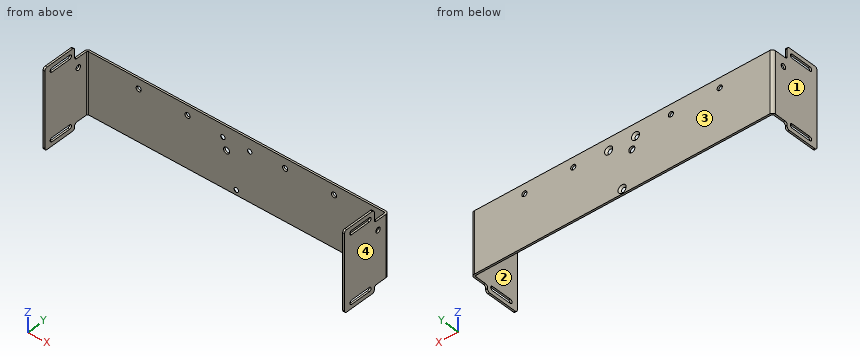
from build123d import *

# Parameters (mm, degrees)
SM_BASE_FLANGE_1_DEPTH       = 50
HOLE_WIZARD_1_AT_2_COUNT     = 2
HOLE_WIZARD_1_AT_2_PITCH     = 37.643060449
HOLE_WIZARD_1_AT_3_COUNT     = 2
HOLE_WIZARD_1_AT_3_PITCH     = 37.643060449
HOLE_WIZARD_4_2_4_2_1_D      = 4.2
HOLE_WIZARD_4_2_4_2_2_REACH  = 257.404
HOLE_WIZARD_4_2_4_2_2_BORE_R = 2.1
HOLE_WIZARD_5_0_5_1_D        = 5
SKETCH_18_W                  = 65
SKETCH_18_H                  = 28
SM_BASE_FLANGE_1_2_DEPTH     = 1.5
HOLE_START                   = -123.5
HOLE_WIZARD_3_4_3_4_2_DEPTH  = 1.5
FILLET_1_R                   = 2
FILLET_1_OF_MIRROR_2_R       = 2


# Read off the part's stored shape, not the designer's step: 基体-法兰1, Ø3.4 (3.4) 直径槽口2
# Sheet-metal steps are written as plain solids
with BuildPart() as part:
    # Sm Base Flange 1 outline → Sm Base Flange 1 (new body)
    with BuildSketch(Plane.XY):
        with BuildLine():
            Line((122, 39), (122, 0))
            Line((122, 0), (123.5, 0))
            Line((123.5, 0), (123.5, 39))
            ThreePointArc((123.5, 39), (122.767766953, 40.767766953), (121, 41.5))
            Line((121, 41.5), (-121, 41.5))
            ThreePointArc((-121, 41.5), (-122.767766953, 40.767766953), (-123.5, 39))
            Line((-123.5, 39), (-123.5, 0))
            Line((-123.5, 0), (-122, 0))
            Line((-122, 0), (-122, 39))
            ThreePointArc((-122, 39), (-121.707106781, 39.707106781), (-121, 40))
            Line((-121, 40), (121, 40))
            ThreePointArc((121, 40), (121.707106781, 39.707106781), (122, 39))
        make_face()
    extrude(amount=SM_BASE_FLANGE_1_DEPTH)

    # 草图9 → 打孔尺寸(%根据)开槽沉头木螺钉的类型1 (revolve, cut)
    with BuildSketch(Plane(origin=(0, 41.5, 4), x_dir=(0, 0, 1), z_dir=(1, 0, 0))):
        Polygon((0, 0), (0, 1.5), (1.7, 1.5), (1.7, 1.6), (3.3, 0), align=None)
    hole_wizard_1 = revolve(axis=Axis((0, 47.85, 4), (0, -1, 0)), mode=Mode.SUBTRACT)

    # 打孔尺寸(%根据)开槽沉头木螺钉的类型1 at 2: 打孔尺寸(%根据)开槽沉头木螺钉的类型1 ×2
    with Locations(*[Vector(-0.29221853559902017, 0, 0.956351571051339) * (i * HOLE_WIZARD_1_AT_2_PITCH) for i in range(1, HOLE_WIZARD_1_AT_2_COUNT)]):
        add(hole_wizard_1, mode=Mode.SUBTRACT)

    # 打孔尺寸(%根据)开槽沉头木螺钉的类型1 at 3: 打孔尺寸(%根据)开槽沉头木螺钉的类型1 ×2
    with Locations(*[Vector(0.2922185355990204, 0, 0.956351571051339) * (i * HOLE_WIZARD_1_AT_3_PITCH) for i in range(1, HOLE_WIZARD_1_AT_3_COUNT)]):
        add(hole_wizard_1, mode=Mode.SUBTRACT)

    # Ø4.2 (4.2) 直径孔1 (through all)
    with Locations(Plane(origin=(0, 41.5, 0), x_dir=(1, 0, 0), z_dir=(0, 1, 0))):
        with Locations((-40, -42), (-80, -42), (40, -42), (80, -42)):
            Hole(HOLE_WIZARD_4_2_4_2_1_D / 2)

    # Ø4.2 (4.2) 直径孔2 bore → Ø4.2 (4.2) 直径孔2 (cut, up to next)
    with BuildSketch(Plane(origin=(123.5, 0, 0), x_dir=(0, 0, -1), z_dir=(1, 0, 0)), mode=Mode.PRIVATE) as hole_wizard_4_2_4_2_2_sk1:
        with Locations((-42, 31.5)):
            Circle(HOLE_WIZARD_4_2_4_2_2_BORE_R)
    hole_wizard_4_2_4_2_2_tool1 = extrude(hole_wizard_4_2_4_2_2_sk1.sketch, amount=-HOLE_WIZARD_4_2_4_2_2_REACH, mode=Mode.PRIVATE) & part.part
    hole_wizard_4_2_4_2_2 = hole_wizard_4_2_4_2_2_tool1.solids().sort_by_distance((123.5, 31.5, 42))[0]
    add(hole_wizard_4_2_4_2_2, mode=Mode.SUBTRACT)

    # 镜向1: Ø4.2 (4.2) 直径孔2 across plane
    add(hole_wizard_4_2_4_2_2.mirror(Plane(origin=(0, 0, 0), x_dir=(0, 0, 1), z_dir=(1, 0, 0))), mode=Mode.SUBTRACT)

    # Ø5.0 (5) 直径孔1 (through all)
    with Locations(Plane(origin=(0, 41.5, 0), x_dir=(1, 0, 0), z_dir=(0, 1, 0))):
        with Locations((-8, -31)):
            Hole(HOLE_WIZARD_5_0_5_1_D / 2)

    # 草图18 → Sm Base Flange 1 2 (add)
    with BuildSketch(Plane.ZY.offset(123.5)):
        with Locations((27.5, 14)):
            Rectangle(SKETCH_18_W, SKETCH_18_H)
    sm_base_flange_1_2 = extrude(amount=-SM_BASE_FLANGE_1_2_DEPTH)

    # Ø3.4 (3.4) 直径槽口2 outline → Ø3.4 (3.4) 直径槽口2 (cut)
    with BuildSketch(Plane.YZ.offset(HOLE_START)):
        with BuildLine():
            ThreePointArc((23.3, 53.3), (25, 55), (23.3, 56.7))
            Line((23.3, 56.7), (6.7, 56.7))
            ThreePointArc((6.7, 56.7), (5, 55), (6.7, 53.3))
            Line((6.7, 53.3), (23.3, 53.3))
        make_face()
        with BuildLine():
            ThreePointArc((23.3, -1.7), (25, 0), (23.3, 1.7))
            Line((23.3, 1.7), (6.7, 1.7))
            ThreePointArc((6.7, 1.7), (5, 0), (6.7, -1.7))
            Line((6.7, -1.7), (23.3, -1.7))
        make_face()
    hole_wizard_3_4_3_4_2 = extrude(amount=HOLE_WIZARD_3_4_3_4_2_DEPTH, mode=Mode.SUBTRACT)

    # 圆角1
    fillet_1_edges = [part.edges().sort_by_distance(p)[0] for p in [
        (-122.75, 28, 0),
        (-122.75, 28, -5),
        (-122.75, 28, 60),
        (-122.75, 0, 60),
        (-122.75, 0, -5),
        (-122.75, 28, 50),
    ]]
    fillet(fillet_1_edges, radius=FILLET_1_R)

    # 镜向2: Sm Base Flange 1 2, Ø3.4 (3.4) 直径槽口2 across plane
    add(sm_base_flange_1_2.mirror(Plane(origin=(0, 0, 0), x_dir=(0, 0, 1), z_dir=(1, 0, 0))))
    add(hole_wizard_3_4_3_4_2.mirror(Plane(origin=(0, 0, 0), x_dir=(0, 0, 1), z_dir=(1, 0, 0))), mode=Mode.SUBTRACT)

    # 圆角1 of 镜向2
    fillet_1_of_mirror_2_edges = [part.edges().sort_by_distance(p)[0] for p in [
        (122.75, 28, 0),
        (122.75, 28, -5),
        (122.75, 28, 60),
        (122.75, 0, 60),
        (122.75, 0, -5),
        (122.75, 28, 50),
    ]]
    fillet(fillet_1_of_mirror_2_edges, radius=FILLET_1_OF_MIRROR_2_R)


solid = part.part
Verification items for the finished model (mm, model axes). Face numbers are marked on the shaded views. Coordinates: 2 decimals unless noted, no trailing zeros. Order: outer loops, then holes, each group sorted by start corner. A loop starts at its lowest first (then second) coordinate and runs counter-clockwise, first axis right, second up. Notation, with made-up numbers: M 36,-29 L 68,-29 A9 ccw 68,-19 Z; hole C -19.5,58.5 d3. An arc over 180 degrees is marked long. One line per item, written item: value. Start each with the question number.
Item 1: Sectioned sample at C-C (z = 12.5). Enter the section's corners in (x, y), then the cut area to 3 significant figures.
Item 2: Sectioned sample at A-A (x = 40). Enter the section's corners in (y, z), then the cut area to 3 significant figures.
Item 3: Gauge pin test, flat ends, axial feed: pin 1 (4 mm diameter, centred on x = -8, z = 31, fed in from +Y); pin 2 (5 mm diameter, centred on x = 80, z = 42, fed in from -Y); pin 3 (0.8 mm diameter, centred on x = -122.5, z = 56.5, fed in from +Y); pin 4 (6 mm diameter, centred on x = -30.5, y = 37.5, fed in from +Z). Record the tip position at first contact, or that the pin passes through.
Item 4: Sectioned sample at D-D (x = 0). Enter the section's corners in (y, z), then the cut area to 4 significant figures.
Item 5: Sectioned sample at B-B (y = 11). Enter the section's corners in (x, z).
Item 6: Scan lines: probe 1 along X at (y, z) = (30, 45); probe 2 along Z at (x, y) = (-40, 40.85); probe 3 along Y at (x, z) = (-64.5, 3). Record each from-to range of solid material in increasing order.
Item 7: Mould release check, pull along X, two halves, no side actions. Record for the marked faces 1, 2, 3 and 4: released by +X, released by -X, zero draft, split by the parting line, or undercut.
Conclusion:
1. outline: M -123.5,0 L -122,0 L -122,39 A1 cw -121,40 L 121,40 A1 cw 122,39 L 122,0 L 123.5,0 L 123.5,39 A2.5 ccw 121,41.5 L -121,41.5 A2.5 ccw -123.5,39 Z
1. area: 488 mm^2
2. outline: M 40,0 L 41.5,0 L 41.5,39.9 L 40,39.9 Z; M 40,44.1 L 41.5,44.1 L 41.5,50 L 40,50 Z
2. area: 68.7 mm^2
3. pin 1: passes through
3. pin 2: stops at y = 40
3. pin 3: stops at y = 28
3. pin 4: stops at z = 50
4. outline: M 40,0 L 41.5,0 L 41.5,0.7 L 40,2.2 Z; M 40,5.8 L 41.5,7.3 L 41.5,50 L 40,50 Z
4. area: 67.35 mm^2
5. outline: M -123.5,-5 L -122,-5 L -122,-1.7 L -123.5,-1.7 Z; M -123.5,1.7 L -122,1.7 L -122,53.3 L -123.5,53.3 Z; M -123.5,56.7 L -122,56.7 L -122,60 L -123.5,60 Z; M 122,-5 L 123.5,-5 L 123.5,-1.7 L 122,-1.7 Z; M 122,1.7 L 123.5,1.7 L 123.5,53.3 L 122,53.3 Z; M 122,56.7 L 123.5,56.7 L 123.5,60 L 122,60 Z
6. probe 1: x = -123.5 to -122, 122 to 123.5
6. probe 2: z = 0 to 39.9, 44.1 to 50
6. probe 3: y = 40 to 41.5
7. face 1: released by -X
7. face 2: undercut
7. face 3: zero draft
7. face 4: released by +X
